Autodesk Inventor part; units mm, degrees
ref_plane "YZ Plane" through (0, 0, 0) normal (1, 0, 0) x (0, 1, 0)
ref_plane "XZ Plane" through (0, 0, 0) normal (0, 1, 0) x (-1, 0, 0)
ref_plane "XY Plane" through (0, 0, 0) normal (0, 0, 1) x (1, 0, 0)
sketch "Sketch1" plane through (0, 0, 0) normal (0, 1, 0) x (-1, 0, 0)
  circle A0 centre (0, 0) radius 10.5
  dimension "d0" = 21
extrude "Extrusion1" add sketch "Sketch1" along normal blind 3
sketch "Sketch2" plane through (0, 3, 0) normal (0, 1, 0) x (1, 0, 0)
  circle A0 centre (0, 0) radius 6
  dimension "d3" = 12
extrude "Extrusion3" add sketch "Sketch2" along normal blind 10
sketch "Sketch4" plane through (0, 13, 0) normal (0, 1, 0) x (1, 0, 0)
  circle A0 centre (0, 0) radius 3
  dimension "d13" = 6
extrude "Extrusion5" cut sketch "Sketch4" against normal through all
chamfer "Chamfer1" distance 3 angle 45 1 edges at (-3, 13, 0)
properties part number "reverse gear lower cylinder ream 1"
The model under review builds one solid part; all positions refer to its coordinate system, in mm. A direction names the side the tool comes from. Round coordinates to 2 decimals unless told otherwise and drop trailing zeros. Write each loop counter-clockwise with the first axis right and the second up, starting at its lowest first coordinate (ties: lowest second). Pieces come first, ordered by that corner, then holes.
(1) Machinability: for faces 4 (the cylindrical face through (-6, 8, 0)), 5 (the flat face through (-2.2, 0, 2.5)), which of the approach directions +Z, -Z, +X, -X, +Y, -Y give a long, thin tool a straight path to every point of the face, cutting with its end or side? Answer none if there is none.
(2) We need section D-D on y = 5.5. Give the boundary of the cut face in (x, z), and give its area (3 significant figures).
(3) Wall thickness on L1, parallel to Z at x = 0, y = 6.75; L2, parallel to Z at x = 0, y = 2.75: over which ranges is each line inside the solid? List them lowest first.
(4) Insertion check: pin 1 (3.5 mm diameter, centred on x = 0, z = 0, fed in from +Y); pin 2 (4 mm diameter, centred on x = 7, y = 3.5, fed in from -Z); pin 3 (4 mm diameter, centred on y = 5.5, z = -5, fed in from -X); pin 4 (4 mm diameter, centred on x = -5, z = -7, fed in from +Y). Each pin has a flat end and moves straight along its axis. Give the tip position at first contact, or say it passes through.
(5) We need section C-C on y = 2. Give the boundary of the cut face in (x, z), and give its area (3 significant figures).
(6) Mouldability with a two-part tool opening along X and no side actions: class faces 1 (the cylindrical face through (-10, 1.5, -3.2)), 2 (the cylindrical face through (-3, 5, 0)), 3 (the flat face through (-5, 3, -5)) as +X half, -X half, draft (parallel to the pull), parting line (faces both ways), or undercut.
Findings below:
1. face 4: +Y
1. face 5: +Z, -Z, +X, -X, -Y
2. outline: circle Ø12 at (0, 0); hole circle Ø6 at (0, 0)
2. area: 84.8 mm2
3. L1: z = -6 to -3, 3 to 6
3. L2: z = -10.5 to -3, 3 to 10.5
4. pin 1: passes through
4. pin 2: stops at z = -9.2
4. pin 3: stops at x = -5.2
4. pin 4: stops at y = 3
5. outline: circle Ø21 at (0, 0); hole circle Ø6 at (0, 0)
5. area: 318 mm2
6. face 1: parting line
6. face 2: undercut
6. face 3: draft
